Read the model definition and answer for the solid it produces. Units are mm, in the model's axes. Face numbers are marked on the shaded views. A direction names the side the tool comes from. Coordinates: 2 decimals unless noted, no trailing zeros. Write each loop counter-clockwise with the first axis right and the second up, starting at its lowest first coordinate (ties: lowest second). Pieces come first, ordered by that corner, then holes.
1) Determine the mould class of the marked faces 1 and 2 for opening direction X: +X half, -X half, draft (parallel to the pull), parting line (faces both ways), or undercut.
2) Which of the six approach directions +Z, -Z, +X, -X, +Y, -Y give full straight-line access (tool end or side, diameter ignored) to the marked faces 3, 4 and 5?
3) Find the intervals of material crossed by line 1 (X direction, y = 21, z = 27); line 2 (X direction, y = 56, z = 24); line 3 (Z direction, x = 15.5, y = 29.5), in increasing order.
4) The part is cut by section D-D (y = 56). Determine the outline of the cut face in (x, z) (1 decimal), then the cut area to 3 significant figures.
5) Each of these flat-tipped pins is pushed along its axis until it touches: pin 1 Ø7 at (y, z) = (62, 9) entering from -X; pin 2 Ø20.5 at (x, y) = (10.5, 46) entering from +Z; pin 3 Ø19.5 at (y, z) = (39.5, 26.5) entering from -X. Where does it stop, or does it pass through?
6) The part is cut by section B-B (x = -19.5). Determine the outline of the cut face in (y, z).
7) The part is cut by section A-A (z = 11). Determine the outline of the cut face in (x, y).
8) The part is cut by section C-C (y = 7.5). Determine the outline of the cut face in (x, z), then the cut area to 3 significant figures.
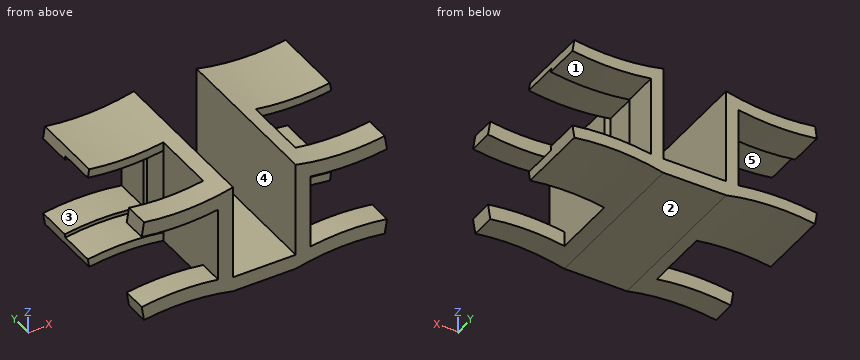
from build123d import *

# Parameters (mm, degrees)
BOSS_EXTRUDE1_DEPTH = 66
CUT_EXTRUDE1_START  = -15
CUT_EXTRUDE1_DEPTH  = 15
CUT_EXTRUDE2_START  = -14.5
CUT_EXTRUDE2_DEPTH  = 15
SKETCH4_W           = 44.566501288
SKETCH4_H           = 26.5
CUT_EXTRUDE3_DEPTH  = 103.576483765
SKETCH5_W           = 44.566501288
SKETCH5_H           = 26.5
CUT_EXTRUDE4_DEPTH  = 103.576483765


with BuildPart() as part:
    # Sketch1 → Boss-Extrude1 (new body)
    with BuildSketch(Plane(origin=(0, 0, 0), x_dir=(1, 0, 0), z_dir=(0, 1, 0))):
        with BuildLine():
            Line((-6, -1.283250644), (-6, -31.283250644))
            ThreePointArc((-6, -31.283250644), (-21.5, -30.074697642), (-37, -31.283250644))
            Line((-37, -31.283250644), (-36.07, -37.210737464))
            ThreePointArc((-36.07, -37.210737464), (-17.969313256, -36.14102822), (0, -38.566501288))
            Line((0, -38.566501288), (0, 0))
            Line((0, 0), (25.4, 0))
            Line((25.4, 0), (25.4, -38.566501288))
            ThreePointArc((25.4, -38.566501288), (43.369313256, -36.14102822), (61.47, -37.210737464))
            Line((61.47, -37.210737464), (62.4, -31.283250644))
            ThreePointArc((62.4, -31.283250644), (46.9, -30.074697642), (31.4, -31.283250644))
            Line((31.4, -31.283250644), (31.4, -1.283250644))
            ThreePointArc((31.4, -1.283250644), (46.9, -2.491803646), (62.4, -1.283250644))
            Line((62.4, -1.283250644), (61.47, 4.644236176))
            ThreePointArc((61.47, 4.644236176), (43.369313256, 3.574526932), (25.4, 6))
            Line((25.4, 6), (0, 6))
            ThreePointArc((0, 6), (-17.969313256, 3.574526932), (-36.07, 4.644236176))
            Line((-36.07, 4.644236176), (-37, -1.283250644))
            ThreePointArc((-37, -1.283250644), (-21.5, -2.491803646), (-6, -1.283250644))
        make_face()
    extrude(amount=BOSS_EXTRUDE1_DEPTH)

    # Sketch2 → Cut-Extrude1 (cut)
    # profile 1 of 2: a face of its own
    with BuildSketch(Plane(origin=(0, 66, 0), x_dir=(1, 0, 0), z_dir=(0, 1, 0)).offset(CUT_EXTRUDE1_START)):
        with BuildLine():
            Line((-5, -0.107120067), (-5, -32.459381221))
            ThreePointArc((-5, -32.459381221), (-21.5, -31.074697642), (-38, -32.459381221))
            Line((-38, -32.459381221), (-38, -0.107120067))
            ThreePointArc((-38, -0.107120067), (-21.5, -1.491803646), (-5, -0.107120067))
        make_face()
        with BuildLine():
            Line((-6, -1.283250644), (-6, -31.283250644))
            ThreePointArc((-6, -31.283250644), (-21.5, -30.074697642), (-37, -31.283250644))
            Line((-37, -31.283250644), (-37, -1.283250644))
            ThreePointArc((-37, -1.283250644), (-21.5, -2.491803646), (-6, -1.283250644))
        make_face(mode=Mode.SUBTRACT)
    # profile 2 of 2: a face of its own
    with BuildSketch(Plane(origin=(0, 66, 0), x_dir=(1, 0, 0), z_dir=(0, 1, 0)).offset(CUT_EXTRUDE1_START)):
        with BuildLine():
            Line((63.4, -0.107120067), (63.4, -32.459381221))
            ThreePointArc((63.4, -32.459381221), (46.9, -31.074697642), (30.4, -32.459381221))
            Line((30.4, -32.459381221), (30.4, -0.107120067))
            ThreePointArc((30.4, -0.107120067), (46.9, -1.491803646), (63.4, -0.107120067))
        make_face()
        with BuildLine():
            Line((31.4, -1.283250644), (31.4, -31.283250644))
            ThreePointArc((31.4, -31.283250644), (46.9, -30.074697642), (62.4, -31.283250644))
            Line((62.4, -31.283250644), (62.4, -1.283250644))
            ThreePointArc((62.4, -1.283250644), (46.9, -2.491803646), (31.4, -1.283250644))
        make_face(mode=Mode.SUBTRACT)
    extrude(amount=CUT_EXTRUDE1_DEPTH, mode=Mode.SUBTRACT)

    # Sketch3 → Cut-Extrude2 (cut)
    # profile 1 of 2: a face of its own
    with BuildSketch(Plane(origin=(0, 51, 0), x_dir=(1, 0, 0), z_dir=(0, 1, 0)).offset(CUT_EXTRUDE2_START)):
        with BuildLine():
            Line((-3.5, 1.684138832), (-3.5, -34.25064012))
            ThreePointArc((-3.5, -34.25064012), (-21.5, -32.574697642), (-39.5, -34.25064012))
            Line((-39.5, -34.25064012), (-39.5, 1.684138832))
            ThreePointArc((-39.5, 1.684138832), (-21.5, 0.008196354), (-3.5, 1.684138832))
        make_face()
        with BuildLine():
            Line((-37, -1.283250644), (-37, -31.283250644))
            ThreePointArc((-37, -31.283250644), (-21.5, -30.074697642), (-6, -31.283250644))
            Line((-6, -31.283250644), (-6, -1.283250644))
            ThreePointArc((-6, -1.283250644), (-21.5, -2.491803646), (-37, -1.283250644))
        make_face(mode=Mode.SUBTRACT)
    # profile 2 of 2: a face of its own
    with BuildSketch(Plane(origin=(0, 51, 0), x_dir=(1, 0, 0), z_dir=(0, 1, 0)).offset(CUT_EXTRUDE2_START)):
        with BuildLine():
            Line((64.9, 1.684138832), (64.9, -34.25064012))
            ThreePointArc((64.9, -34.25064012), (46.9, -32.574697642), (28.9, -34.25064012))
            Line((28.9, -34.25064012), (28.9, 1.684138832))
            ThreePointArc((28.9, 1.684138832), (46.9, 0.008196354), (64.9, 1.684138832))
        make_face()
        with BuildLine():
            Line((31.4, -1.283250644), (31.4, -31.283250644))
            ThreePointArc((31.4, -31.283250644), (46.9, -30.074697642), (62.4, -31.283250644))
            Line((62.4, -31.283250644), (62.4, -1.283250644))
            ThreePointArc((62.4, -1.283250644), (46.9, -2.491803646), (31.4, -1.283250644))
        make_face(mode=Mode.SUBTRACT)
    extrude(amount=CUT_EXTRUDE2_DEPTH, mode=Mode.SUBTRACT)

    # Sketch4 → Cut-Extrude3 (cut, through all)
    with BuildSketch(Plane.ZY.offset(6)):
        with Locations((16.283250644, 23.25)):
            Rectangle(SKETCH4_W, SKETCH4_H)
    extrude(amount=CUT_EXTRUDE3_DEPTH, mode=Mode.SUBTRACT)

    # Sketch5 → Cut-Extrude4 (cut, through all)
    with BuildSketch(Plane(origin=(31.4, 0, 0), x_dir=(0, 0, -1), z_dir=(1, 0, 0))):
        with Locations((-16.283250644, 23.25)):
            Rectangle(SKETCH5_W, SKETCH5_H)
    extrude(amount=CUT_EXTRUDE4_DEPTH, mode=Mode.SUBTRACT)


solid = part.part
Reported:
1. face 1: undercut
1. face 2: draft
2. face 3: +Y
2. face 4: +Z, +Y, -Y
2. face 5: none
3. line 1: x = -6 to 0, 25.4 to 31.4
3. line 2: x = -5 to 0, 25.4 to 30.4
3. line 3: z = -6 to 0
4. outline: (-36.8, 0.3) - (-36.1, -4.6) arc R94 cw to (0, -6) - (25.4, -6) arc R94 cw to (61.5, -4.6) - (62.2, 0.3) arc R99 ccw to (30.4, 0.1) - (30.4, 32.5) arc R99 ccw to (62.2, 32.3) - (61.5, 37.2) arc R94 cw to (25.4, 38.6) - (25.4, 0) - (0, 0) - (0, 38.6) arc R94 cw to (-36.1, 37.2) - (-36.8, 32.3) arc R99 ccw to (-5, 32.5) - (-5, 0.1) arc R99 ccw to start
4. area: 1,220 mm2
5. pin 1: stops at x = -5
5. pin 2: stops at z = 0
5. pin 3: stops at x = -36.61
6. outline: (0, -3.53) - (10, -3.53) - (10, 2.47) - (0, 2.47) - close; (0, 30.09) - (10, 30.09) - (10, 36.1) - (0, 36.1) - close; (36.5, -3.53) - (66, -3.53) - (66, 1.47) - (51.5, 1.47) - (51.5, -0.03) - (36.5, -0.03) - close; (36.5, 32.6) - (51.5, 32.6) - (51.5, 31.09) - (66, 31.09) - (66, 36.1) - (36.5, 36.1) - close
7. outline: (-6, 0) - (0, 0) - (0, 66) - (-5, 66) - (-5, 51.5) - (-3.5, 51.5) - (-3.5, 36.5) - (-6, 36.5) - close; (25.4, 0) - (31.4, 0) - (31.4, 36.5) - (28.9, 36.5) - (28.9, 51.5) - (30.4, 51.5) - (30.4, 66) - (25.4, 66) - close
8. outline: (-37, 1.28) - (-36.07, -4.64) arc R94 cw to (0, -6) - (25.4, -6) arc R94 cw to (61.47, -4.64) - (62.4, 1.28) arc R100 ccw to (31.4, 1.28) - (31.4, 31.28) arc R100 ccw to (62.4, 31.28) - (61.47, 37.21) arc R94 cw to (25.4, 38.57) - (25.4, 0) - (0, 0) - (0, 38.57) arc R94 cw to (-36.07, 37.21) - (-37, 31.28) arc R100 ccw to (-6, 31.28) - (-6, 1.28) arc R100 ccw to start
8. area: 1,410 mm2
